from build123d import *

# Parameters (mm, degrees)
F2_W     = 73.8781243563
F2_H     = 160.1297496091
F2_W_2   = 40
F2_H_2   = 126.2516252528
F3_DEPTH = 25
F4_R     = 2.75
F5_DEPTH = 25
F6_SIZE  = 1


with BuildPart() as f1:
    # F0 (on Right) → F1 (revolve)
    with BuildSketch(Plane.YZ):
        Polygon((10, 24), (0, 24), (0, 8), (57, 8), (57, 14), (10, 14), align=None)
    revolve(axis=Axis((0, 17.6531788457, 0), (0, 1, 0)))

    # F2 (on face) → F3 (cut)
    with BuildSketch(Plane.XZ):
        Rectangle(F2_W, F2_H)
        Rectangle(F2_W_2, F2_H_2, mode=Mode.SUBTRACT)
    extrude(amount=-F3_DEPTH, mode=Mode.SUBTRACT)

    # F4 (on face) → F5 (cut)
    with BuildSketch(Plane.XZ):
        with Locations((0, 19)):
            Circle(F4_R)
        with Locations((-13.4350288425, 13.4350288425)):
            Circle(F4_R)
        with Locations((-13.4350288425, -13.4350288425)):
            Circle(F4_R)
        with Locations((0, -19)):
            Circle(F4_R)
        with Locations((13.4350288425, -13.4350288425)):
            Circle(F4_R)
        with Locations((13.4350288425, 13.4350288425)):
            Circle(F4_R)
    extrude(amount=-F5_DEPTH, mode=Mode.SUBTRACT)

    # F6
    f6_edges = [f1.edges().sort_by_distance(p)[0] for p in [
        (0, 0, -8),
        (0, 57, -8),
        (0, 28.5, 8),
        (0, 57, -14),
        (0, 0, 24),
        (0, 0, -24),
        (0, 10, 24),
        (0, 10, -24),
    ]]
    chamfer(f6_edges, length=F6_SIZE)


solid = f1.part
For this review, take the finished solid that the model builds, in its own axes (mm). A direction names the side the tool comes from. Give positions to 0.01 mm unless a question says otherwise; leave off trailing zeros. Order: outer loops, then holes, each group sorted by start corner. A loop starts at its lowest first (then second) coordinate and runs counter-clockwise, first axis right, second up. Notation, with made-up numbers: (22, -25) - (54, -25) arc R22 cw to (54, -3) - close; hole circle Ø3 at (55.25, 44.25). An arc over 180 degrees is marked (long way). Answer as a JSON object with one key per item and string values. Group by question number.
Item 1: Take a section at A-A on x = 0. Give the number of separate pieces and of enclosed holes in the cut face, and give its area (3 significant figures).
Item 2: Machinability: for faces 5 (the flat face through (9, 57, -3)), 6 (the cylindrical face through (-5.362, 32.678, 12.932)), which of the approach directions +Z, -Z, +X, -X, +Y, -Y give a long, thin tool a straight path to every point of the face, cutting with its end or side? Answer none if there is none.
Item 3: Clearance check with flat-ended pins moving along their axes: pin 1 Ø9 at (x, z) = (-13.44, 13.44) entering from +Y; pin 2 Ø1.5 at (x, y) = (7, 15.5) entering from -Z; pin 3 Ø6 at (y, z) = (47, -0.5) entering from -X. State where each tip first meets the part, or that it passes through.
Item 4: Take a section at B-B on z = 0. Give the boundary of the cut face in (x, y), and give its area (3 significant figures).
Item 5: Take a section at C-C on y = 25.5. Give the boundary of the cut face in (x, z), and give its area (3 significant figures).
Item 6: Draft analysis for pull direction X (two halves, no side actions). For faces 1 (the flat face through (-20, 5, 0)), 2 (the flat face through (14, 10, 5)), 3 (the conical face through (-0.3, 0.2, 23.2)), 4 (the cylindrical face through (-7.81, 28.88, -1.73)), state which applies: pulls with the +X half, pulls with the -X half, needs draft (parallel to the pull), parting line crosses it, or undercut.
Item 7: Wall thickness on line 1 along Y through (x, z) = (12, -18.5); line 2 along X through (y, z) = (49.5, -2); line 3 along X through (y, z) = (22, -5) (3 decimals): over which ranges is each line inside the solid? List them lowest first.
Reported:
{
 "1": {"separate pieces": "4", "enclosed holes": "0", "area": "769 mm^2"},
 "2": {"face 5": "+Z, -Z, +X, -X, +Y", "face 6": "+Y"},
 "3": {"pin 1": "y = 10", "pin 2": "z = -12.53", "pin 3": "x = -14"},
 "4": {"outline": "(-20, 0) - (-9, 0) - (-8, 1) - (-8, 56) - (-9, 57) - (-13, 57) - (-14, 56) - (-14, 10) - (-20, 10) - close; (8, 1) - (9, 0) - (20, 0) - (20, 10) - (14, 10) - (14, 56) - (13, 57) - (9, 57) - (8, 56) - close", "area": "801 mm^2"},
 "5": {"outline": "circle Ø28 at (0, 0); hole circle Ø16 at (0, 0)", "area": "415 mm^2"},
 "6": {"face 1": "pulls with the -X half", "face 2": "needs draft", "face 3": "parting line crosses it", "face 4": "undercut"},
 "7": {"line 1": "0 to 10", "line 2": "-13.86 to -7.75, 7.75 to 13.86", "line 3": "-13.077 to -6.245, 6.245 to 13.077"}
}
